from build123d import *

# Parameters (mm, degrees)
F2_T     = -6
F4_W     = 30
F4_H     = 50
F6_R     = 3
F7_DEPTH = 2


# Not quite as in the source:
# - a pattern or mirror of a feature is missing from the dataset's text; its kind, count and spacing are read off the source's solid


with BuildPart() as f1:
    # F0 (on Front) → F1 (revolve)
    with BuildSketch(Plane.XZ):
        with BuildLine():
            Line((0, 50), (-86.6025403784, 50))
            ThreePointArc((-86.6025403784, 50), (-96.5925826289, 25.8819045103), (-100, 0))
            Line((-100, 0), (0, 0))
            Line((0, 0), (0, 50))
        make_face()
    revolve(axis=Axis((0, 0, 25), (0, 0, -1)))

    # F2
    f2_openings = [f1.faces().sort_by_distance(p)[0] for p in [
        (0, 0, 50),
        (0, 0, 0),
    ]]
    offset(amount=F2_T, openings=f2_openings)

    # F4 (on offset) → F5 (join, up to the next surface of F1)
    with BuildSketch(Plane.XZ.offset(-60)):
        with Locations((0, 25)):
            Rectangle(F4_W, F4_H)
    f5 = extrude(until=Until.NEXT, dir=(0, 1, 0))

    # F5_copies: F5 across plane
    add(f5.mirror(Plane(origin=(0, 0, 0), x_dir=(0, 0, -1), z_dir=(0, -1, 0))))

    # F6 (on face) → F7 (cut)
    with BuildSketch(Plane.XZ.offset(-60)):
        with Locations((0, 25)):
            Circle(F6_R)
    f7 = extrude(amount=-F7_DEPTH, mode=Mode.SUBTRACT)

    # F7_copies: F7 across plane
    add(f7.mirror(Plane(origin=(0, 0, 0), x_dir=(0, 0, -1), z_dir=(0, -1, 0))), mode=Mode.SUBTRACT)


solid = f1.part
Build history of the part. All positions in model axes, mm. A direction names the side the tool comes from. Give positions to 0.01 mm unless a question says otherwise; leave off trailing zeros. Loops run counter-clockwise (first coordinate to the right, second up) from the corner with the lowest first, then second, coordinate; pieces in that order, holes last. Notation, with made-up numbers: (52.25, 88) - (102.25, 88) arc R13 ccw to (102.25, 106) - close; hole circle Ø1 at (-26.5, 36.25). An arc over 180 degrees is marked (long way). Write item = value, one per line. Start each with the question number.
1) Band-saw the part on C-C on z = 25. Give the cut face in (x, y), plus the area to 3 significant figures.
2) Pull direction Y, two halves, no side cores. Call faces 1 (the flat face through (0, 67, 0)), 2 (the cylindrical face through (-0.65, 60.99, 22.07)): +Y half, -Y half, draft (parallel to the pull), parting line (faces both ways), or undercut.
3) Band-saw the part on A-A on x = 0. Give the cut face in (y, z).
4) Tool access for faces 3 (the flat face through (15, 76, 25)), 4 (the flat face through (-4, -60, 25)), 5 (the cylindrical face through (-0.65, -60.99, 22.07)): list every direction of +Z, -Z, +X, -X, +Y, -Y with a clear straight run to the whole face (end or side of a thin tool).
5) Band-saw the part on B-B on y = -6. Give the cut face in (x, z).
6) Drop flat-ended pins along their axis: pin 1 Ø3.5 at (x, z) = (0, 25) entering from -Y; pin 2 Ø3 at (x, z) = (60, 30.5) entering from -Y; pin 3 Ø4 at (y, z) = (69.5, 15.5) entering from +X. Give the stop position or say it passes through.
7) Band-saw the part on D-D on y = -73. Give the cut face in (x, z).
8) Probe probe 1 along Z at (x, y) = (0, -60.85); probe 2 along X at (y, z) = (-69.5, 37.5); probe 3 along X at (y, z) = (34, 14). List the from-to ranges inside material, lowest first. Write a range as from..to.
Final values:
q1.outline = circle Ø193.65 at (0, 0); hole (-15, -89.36) - (-15, -60) - (-3, -60) - (-3, -62) - (3, -62) - (3, -60) - (15, -60) - (15, -89.36) arc R90.61 ccw to (15, 89.36) - (15, 60) - (3, 60) - (3, 62) - (-3, 62) - (-3, 60) - (-15, 60) - (-15, 89.36) arc R90.61 ccw to start
q1.area = 5,440 mm²
q2.face_1 = draft
q2.face_2 = undercut
q3.outline = (-100, 0) - (-60, 0) - (-60, 22) - (-62, 22) - (-62, 28) - (-60, 28) - (-60, 50) - (-86.6, 50) arc R100 ccw to start; (60, 0) - (100, 0) arc R100 ccw to (86.6, 50) - (60, 50) - (60, 28) - (62, 28) - (62, 22) - (60, 22) - close
q4.face_3 = -Z
q4.face_4 = +Z, -Z
q4.face_5 = none
q5.outline = (-99.82, 0) - (-93.81, 0) arc R93.81 cw to (-79.37, 50) - (-86.39, 50) arc R99.82 ccw to start; (79.37, 50) arc R93.81 cw to (93.81, 0) - (99.82, 0) arc R99.82 ccw to (86.39, 50) - close
q6.pin_1 = -97.26
q6.pin_2 = -75.3
q6.pin_3 = 72.18
q7.outline = (-68.34, 0) - (-59.22, 0) arc R59.22 cw to (-31.73, 50) - (-46.59, 50) arc R68.34 ccw to start; (-15, 0) - (15, 0) - (15, 50) - (-15, 50) - close; (31.73, 50) arc R59.22 cw to (59.22, 0) - (68.34, 0) arc R68.34 ccw to (46.59, 50) - close
q8.probe_1 = 0..22, 28..50
q8.probe_2 = -61.35..-50.99, -15..15, 50.99..61.35
q8.probe_3 = -92.99..-86.51, 86.51..92.99
